Geometry check sheet. Reference: the model listing, model coordinates, mm. A direction names the side the tool comes from. Coordinates: 2 decimals unless noted, no trailing zeros. Loops run counter-clockwise (first coordinate to the right, second up) from the corner with the lowest first, then second, coordinate; pieces in that order, holes last. Notation, with made-up numbers: M -32,33 L 21,33 A26 ccw 21,70 Z; hole C -19.5,59 d8. An arc over 180 degrees is marked long. Use CSV: the item, a comma, the result in double quotes.
```python
from build123d import *

# Parameters (mm, degrees)
BOSS_EXTRUDE1_DEPTH      = 5
BOSS_EXTRUDE1_DEPTH_BACK = 13
SKETCH2_R                = 1.5
CUT_EXTRUDE1_DEPTH       = 66.915554427
SKETCH3_R                = 2
CUT_EXTRUDE2_DEPTH       = 68.080998169
SKETCH4_W                = 8
SKETCH4_H                = 4.7
BOSS_EXTRUDE2_DEPTH      = 6


with BuildPart() as part:
    # Sketch1 → Boss-Extrude1 (new, two sides: drawn at the far end of the back side and taken through both)
    with BuildSketch(Plane.XY.offset(-BOSS_EXTRUDE1_DEPTH_BACK)):
        Polygon((0, 6), (5, 6), (5, -5), (-13.675831366, -17.768137002), (-49.056349186, -22.556349186), (-60.556349186, -11.056349186), (-46.414213562, 3.085786438), (-34.328427125, -9), (-21.164213562, -9), (-8, 0), (0, 0), align=None)
    extrude(amount=BOSS_EXTRUDE1_DEPTH + BOSS_EXTRUDE1_DEPTH_BACK)

    # Sketch2 → Cut-Extrude1 (cut, through all)
    with BuildSketch(Plane(origin=(0, 0, 0), x_dir=(1, 0, 0), z_dir=(0, 1, 0))):
        with Locations(Location((-3, 3.95, 0), (0, 0, 270))):
            Circle(SKETCH2_R)
    extrude(amount=-CUT_EXTRUDE1_DEPTH, mode=Mode.SUBTRACT)

    # Sketch3 → Cut-Extrude2 (cut, through all)
    with BuildSketch(Plane(origin=(0, 0, -13), x_dir=(-1, 0, 0), z_dir=(0, 0, -1))):
        with Locations((50.475737372, -12.65147749)):
            Circle(SKETCH3_R)
        with Locations((44.701932157, -7.111978477)):
            Circle(SKETCH3_R)
    extrude(amount=-CUT_EXTRUDE2_DEPTH, mode=Mode.SUBTRACT)

    # Sketch4 → Boss-Extrude2 (add)
    with BuildSketch(Plane(origin=(0, 0, 0), x_dir=(1, 0, 0), z_dir=(0, 1, 0))):
        with Locations((-4, -2.65)):
            Rectangle(SKETCH4_W, SKETCH4_H)
        with Locations((-4, 10.65)):
            Rectangle(SKETCH4_W, SKETCH4_H)
    extrude(amount=BOSS_EXTRUDE2_DEPTH)


solid = part.part
```
1. Set-up check for faces 1 (the flat face through (-54.726, -16.887, -4.126)), 2 (the flat face through (-4, 3, 0.3)), 3 (the flat face through (-40.46, -2.87, -4.13)): record each of +Z, -Z, +X, -X, +Y, -Y from which the full face is reachable in a straight line by a thin tool's end or side.
The answers:
face 1,"+Z, -Z, -X, -Y"
face 2,"+Y"
face 3,"+Z, -Z, +Y"
2. Section check A-A, the plane y = -2.75. Record the cut outline in (x, z).
The answers:
outline,"M -52.25,-13 L -40.58,-13 L -40.58,5 L -52.25,5 Z; M -12.02,-13 L 5,-13 L 5,5 L -12.02,5 Z; hole C -3,-3.95 d3"
3. Gauge pin test, flat ends, axial feed: P1, Ø4, axis at y = 4.5, z = 2, coming from the -X side; P2, Ø6, axis at x = -53, z = -4.5, coming from the -Y side; P3, Ø3, axis at y = 2.5, z = -6, coming from the -X side; P4, Ø5, axis at x = -50.48, y = -12.65, coming from the +Z side. Record the tip position at first contact, or that the pin passes through.
The answers:
P1,"x = -47"
P2,"y = -21.61"
P3,"x = -48.5"
P4,"z = 5"
4. Section check B-B, the plane z = -3.95. Record the cut outline in (x, y).
The answers:
outline,"M -60.56,-11.06 L -49.06,-22.56 L -13.68,-17.77 L -4.5,-11.49 L -4.5,0 L -8,0 L -21.16,-9 L -34.33,-9 L -46.41,3.09 Z; M -1.5,-9.44 L 5,-5 L 5,6 L 0,6 L 0,0 L -1.5,0 Z; hole C -50.48,-12.65 d4; hole C -44.7,-7.11 d4"
5. Thickness scan on line 1 (X direction, y = -6.25, z = 2.25); line 2 (Z direction, x = -3, y = -3.5); line 3 (X direction, y = -7, z = -3.95). Record the ranges inside material, lowest first. Write a range as [from, to].
The answers:
line 1,"[-55.75, -46.51], [-42.9, -37.08], [-17.14, 3.17]"
line 2,"[-13, -5.45], [-2.45, 5]"
line 3,"[-56.5, -46.7], [-42.71, -36.33], [-18.24, -4.5], [-1.5, 2.07]"
6. Section check C-C, the plane x = -3. Record the cut outline in (y, z).
The answers:
outline,"M -10.47,-13 L 6,-13 L 6,-8.3 L 0,-8.3 L 0,-5.45 L -10.47,-5.45 Z; M -10.47,-2.45 L 0,-2.45 L 0,0.3 L 6,0.3 L 6,5 L -10.47,5 Z"
7. Release check for a two-part mould opening along X. For faces 4 (the flat face through (1, 6, -4)), 5 (the flat face through (-4, 3, -8.3)), 6 (the flat face through (-31.12, -20.13, -4.13)) record: +X half, -X half, draft (parallel to the pull), parting line (faces both ways), or undercut.
The answers:
face 4,"draft"
face 5,"undercut"
face 6,"+X half"
8. Section check D-D, the plane y = -6. Record the cut outline in (x, z).
The answers:
outline,"M -55.5,-13 L -46.36,-13 L -46.36,5 L -55.5,5 Z; M -43.04,-13 L -37.33,-13 L -37.33,5 L -43.04,5 Z; M -16.78,-13 L 3.54,-13 L 3.54,5 L -16.78,5 Z; hole C -3,-3.95 d3"
